```python
from build123d import *

# Parameters (mm, degrees)
F0_W       = 8
F0_H       = 4
F1_DEPTH   = 110
F2_W       = 8
F2_H       = 4
F3_DEPTH   = 25
F4_R       = 2
F5_DEPTH   = 55.001
F6_R       = 3
F7_SIZE2   = 2
F7_SIZE    = 3
F7_2_SIZE2 = 2
F7_2_SIZE  = 3
F8_R       = 3
F9_R       = 0.7


with BuildPart() as f1:
    # F0 (on Top) → F1 (new body)
    with BuildSketch(Plane.XY):
        with Locations((3.6675264128, -2.3501528167)):
            Rectangle(F0_W, F0_H)
    extrude(amount=F1_DEPTH)

    # F2 (on face) → F3 (join)
    with BuildSketch(Plane(origin=(0, -0.3501528167, 0), x_dir=(-1, 0, 0), z_dir=(0, 1, 0))):
        with Locations((-3.6675264128, 53)):
            Rectangle(F2_W, F2_H)
    extrude(amount=F3_DEPTH)

    # F4 (on face) → F5 (cut, through all)
    with BuildSketch(Plane.XY.offset(55)):
        with Locations((3.6675264128, 19.6498471833)):
            Circle(F4_R)
    extrude(amount=-F5_DEPTH, mode=Mode.SUBTRACT)

    # F6
    f6_edges = [f1.edges().sort_by_distance(p)[0] for p in [
        (3.667526, -0.350153, 55),
        (3.667526, -0.350153, 51),
    ]]
    fillet(f6_edges, radius=F6_R)

    # F7
    f7_edges = [f1.edges().sort_by_distance(p)[0] for p in [
        (7.667526, -4.350153, 55),
    ]]
    f7_side = f1.faces().sort_by_distance((7.667526, 0.334925, 54.618055))[0]
    chamfer(f7_edges, length=F7_SIZE, length2=F7_SIZE2, reference=f7_side)

    # F7#2
    f7_2_edges = [f1.edges().sort_by_distance(p)[0] for p in [
        (-0.332474, -4.350153, 55),
    ]]
    f7_2_side = f1.faces().sort_by_distance((-0.332474, 0.334925, 54.618055))[0]
    chamfer(f7_2_edges, length=F7_2_SIZE, length2=F7_2_SIZE2, reference=f7_2_side)

    # F8
    f8_edges = [f1.edges().sort_by_distance(p)[0] for p in [
        (7.667526, 24.649847, 53),
        (-0.332474, 24.649847, 53),
    ]]
    fillet(f8_edges, radius=F8_R)

    # F9
    f9_edges = [f1.edges().sort_by_distance(p)[0] for p in [
        (-0.332474, 12.149847, 51),
        (-0.332474, 21.649847, 53),
        (-0.332474, 0.528527, 50.12132),
        (-0.332474, 12.149847, 55),
        (-0.332474, -0.350153, 24),
        (-0.332474, 0.528527, 55.87868),
        (-0.332474, -0.850153, 0),
        (-0.332474, -0.350153, 84),
        (-0.332474, -1.350153, 55),
        (-0.332474, -0.850153, 110),
        (7.667526, 12.149847, 55),
        (7.667526, 21.649847, 53),
        (7.667526, 0.528527, 55.87868),
        (7.667526, 12.149847, 51),
        (7.667526, -0.350153, 84),
        (7.667526, 0.528527, 50.12132),
        (7.667526, -0.850153, 110),
        (7.667526, -0.350153, 24),
        (7.667526, -1.350153, 55),
        (7.667526, -0.850153, 0),
        (3.667526, -4.350153, 110),
        (0.667526, -2.850153, 110),
        (6.667526, -2.850153, 110),
        (3.667526, -0.350153, 110),
        (3.667526, -4.350153, 0),
        (0.667526, -2.850153, 0),
        (6.667526, -2.850153, 0),
        (3.667526, -0.350153, 0),
        (1.667526, -4.350153, 55),
        (5.667526, -4.350153, 55),
    ]]
    fillet(f9_edges, radius=F9_R)


solid = f1.part
```
The listing builds one solid part. Answer for the finished solid, in the listing's coordinates (mm). A direction names the side the tool comes from. Coordinates: 2 decimals unless noted, no trailing zeros. Loops run counter-clockwise (first coordinate to the right, second up) from the corner with the lowest first, then second, coordinate; pieces in that order, holes last. Notation, with made-up numbers: (11.5, 36) - (67.5, 36) arc R11 cw to (67.5, 53) - close; hole circle Ø9 at (-19.5, 89). An arc over 180 degrees is marked (long way). Use a Markdown table: item, result. Add a question column.
1) The part is cut by section A-A, the plane z = 17.5. Give the vertices of the cut face in (x, y).
2) Find the intervals of material crossed by line 1 (Z direction, x = 3, y = 11.25); line 2 (Y direction, x = 3.5, z = 42), in increasing order.
3) The part is cut by section B-B, the plane y = 5. Give the vertices of the cut face in (x, z), and give its area (3 significant figures).
4) Given pin 1 (3 mm diameter, centred on x = 6.5, z = 51, fed in from -Y); pin 2 (2 mm diameter, centred on x = 2, y = 17, fed in from -Z); pin 3 (3.5 mm diameter, centred on x = 4.5, y = 16, fed in from +Z); pin 4 (3.5 mm diameter, centred on x = 5, z = 81.5, fed in from +Y), each flat-ended and moving along its own axis, determine where each tip first touches the part or whether it passes through.
5) For faces 1 (the flat face through (4, 13, 55)), 2 (the cylindrical face through (6.53, -2.68, 0.2)), 3 (the flat face through (4, 13, 51)), determine the directions among +Z, -Z, +X, -X, +Y, -Y from which every point of the face is accessible in a straight line to the end or side of a thin tool.
6) The mould has two halves that part along X. Classify faces 4 (the cylindrical face through (6.53, -2.68, 109.8)), 5 (the cylindrical face through (3.23, 17.7, 53.03)), 6 (the flat face through (4, -0.35, 83)): released by +X, released by -X, zero draft, split by the parting line, or undercut.
Here are the results:
| question | item | result |
|---|---|---|
| 1 | outline | (-0.33, -1.14) arc R0.7 ccw to (-0.21, -1.53) - (1.46, -4.04) arc R0.7 ccw to (2.04, -4.35) - (5.29, -4.35) arc R0.7 ccw to (5.88, -4.04) - (7.55, -1.53) arc R0.7 ccw to (7.67, -1.14) - (7.67, -1.05) arc R0.7 ccw to (6.97, -0.35) - (0.37, -0.35) arc R0.7 ccw to (-0.33, -1.05) - close |
| 2 | line 1 | z = 51 to 55 |
| 2 | line 2 | y = -4.35 to -0.35 |
| 3 | outline | (-0.33, 51.7) arc R0.7 ccw to (0.37, 51) - (6.97, 51) arc R0.7 ccw to (7.67, 51.7) - (7.67, 54.3) arc R0.7 ccw to (6.97, 55) - (0.37, 55) arc R0.7 ccw to (-0.33, 54.3) - close |
| 3 | area | 31.6 mm^2 |
| 4 | pin 1 | stops at y = -4.35 |
| 4 | pin 2 | stops at z = 51 |
| 4 | pin 3 | stops at z = 55 |
| 4 | pin 4 | stops at y = -0.35 |
| 5 | face 1 | +Z, +X, -X, +Y |
| 5 | face 2 | -Z, +X, -Y |
| 5 | face 3 | -Z, +X, -X, +Y |
| 6 | face 4 | released by +X |
| 6 | face 5 | undercut |
| 6 | face 6 | zero draft |
